For this review, take the finished solid that the model builds, in its own axes (mm). Round coordinates to 2 decimals unless told otherwise and drop trailing zeros. Order: outer loops, then holes, each group sorted by start corner. A loop starts at its lowest first (then second) coordinate and runs counter-clockwise, first axis right, second up. Notation, with made-up numbers: (50, 6) - (106, 6) arc R32 ccw to (106, 32) - close; hole circle Ø1 at (24.25, -31.5). An arc over 180 degrees is marked (long way). Write each question's results on one line, items separated by ' | '. Start each with the question number.
(1) Take a section at A-A, the plane z = 8. Give the boundary of the cut face in (x, y) (3 decimals), plus the area to 3 significant figures.
(2) Take a section at C-C, the plane y = 1.75. Give the boundary of the cut face in (x, z) (3 decimals), plus the area to 3 significant figures.
(3) Take a section at B-B, the plane x = 22. Give the boundary of the cut face in (y, z) (3 decimals).
(4) Draft analysis for pull direction Z (two halves, no side actions). For faces 1 (the flat face through (-59, 1, 0)), 2 (the flat face through (-64, 0, 0)), state which applies: pulls with the +Z half, pulls with the -Z half, needs draft (parallel to the pull), parting line crosses it, or undercut.
(5) For L1, parallel to Z at x = 47, y = 2.25 (3 decimals); L2, parallel to X at y = 0.85, z = 84.5 (3 decimals); L3, parallel to X at y = 2.6, z = 78 (3 decimals), list the stretches that pass through material, from the lowest coordinate up. Write a range as from..to.
```python
from build123d import *

# Parameters (mm, degrees)
SKETCH_1_W          = 131.75
SKETCH_1_H          = 199.75
EXTRUDE_1_DEPTH     = 3
SKETCH_2_W          = 111.75
SKETCH_2_H          = 179.75
CUT_EXTRUDE_1_DEPTH = 6
SKETCH_3_W          = 121.75
SKETCH_3_H          = 189.75
CUT_EXTRUDE_2_DEPTH = 1


with BuildPart() as part:
    # Эскиз1 → Бобышка-Вытянуть1 (new body)
    with BuildSketch(Plane(origin=(0, 0, 0), x_dir=(1, 0, 0), z_dir=(0, 1, 0))):
        Rectangle(SKETCH_1_W, SKETCH_1_H)
    extrude(amount=EXTRUDE_1_DEPTH)

    # Эскиз2 → Вырез-Вытянуть1 (cut)
    with BuildSketch(Plane(origin=(0, 3, 0), x_dir=(1, 0, 0), z_dir=(0, 1, 0))):
        Rectangle(SKETCH_2_W, SKETCH_2_H)
    extrude(amount=-CUT_EXTRUDE_1_DEPTH, mode=Mode.SUBTRACT)

    # Эскиз3 → Вырез-Вытянуть2 (cut)
    with BuildSketch(Plane.XZ):
        Rectangle(SKETCH_3_W, SKETCH_3_H)
    extrude(amount=-CUT_EXTRUDE_2_DEPTH, mode=Mode.SUBTRACT)


solid = part.part
```
Results below:
1) outline: (-65.875, 0) - (-60.875, 0) - (-60.875, 1) - (-55.875, 1) - (-55.875, 3) - (-65.875, 3) - close; (55.875, 1) - (60.875, 1) - (60.875, 0) - (65.875, 0) - (65.875, 3) - (55.875, 3) - close | area: 50.0 mm^2
2) outline: (-65.875, -99.875) - (65.875, -99.875) - (65.875, 99.875) - (-65.875, 99.875) - close; hole (-55.875, -89.875) - (55.875, -89.875) - (55.875, 89.875) - (-55.875, 89.875) - close | area: 6,230 mm^2
3) outline: (0, -99.875) - (3, -99.875) - (3, -89.875) - (1, -89.875) - (1, -94.875) - (0, -94.875) - close; (0, 94.875) - (1, 94.875) - (1, 89.875) - (3, 89.875) - (3, 99.875) - (0, 99.875) - close
4) face 1: undercut | face 2: needs draft
5) L1: z = -99.875..-89.875, 89.875..99.875 | L2: x = -65.875..-60.875, 60.875..65.875 | L3: x = -65.875..-55.875, 55.875..65.875
